The listing builds one solid part. Answer for the finished solid, in the listing's coordinates (mm). A direction names the side the tool comes from. Coordinates: 2 decimals unless noted, no trailing zeros. Write each loop counter-clockwise with the first axis right and the second up, starting at its lowest first coordinate (ties: lowest second). Pieces come first, ordered by that corner, then holes. Notation, with made-up numbers: M 3,80.5 L 53,80.5 A28 cw 53,100.5 Z; hole C 6,-23.5 d5. An arc over 180 degrees is marked long. Answer as CSV lines item,"result".
Autodesk Inventor part; units mm, degrees
ref_plane "YZ Plane" through (0, 0, 0) normal (1, 0, 0) x (0, 1, 0)
ref_plane "XZ Plane" through (0, 0, 0) normal (0, 1, 0) x (-1, 0, 0)
ref_plane "XY Plane" through (0, 0, 0) normal (0, 0, 1) x (1, 0, 0)
sketch "Sketch1" plane through (0, 0, 0) normal (1, 0, 0) x (0, 1, 0)
  line L0 (-4, 6) -> (-4, -6)
  line L1 (-4, -6) -> (-2, -6)
  line L2 (2, -6) -> (4, -6)
  line L3 (4, -6) -> (4, 6)
  line L4 (4, 6) -> (2, 6)
  line L5 (2, 6) -> (0.5, 2)
  line L6 (0.5, 2) -> (-0.5, 2)
  line L7 (-0.5, 2) -> (-2, 6)
  line L8 (-2, 6) -> (-4, 6)
  line L9 (2, -6) -> (0.5, -2)
  line L10 (0.5, -2) -> (-0.5, -2)
  line L11 (-0.5, -2) -> (-2, -6)
  point P0 (0, 0)
  point P1 (-4, 0)
  point P2 (4, 0)
  point P3 (0, 2)
  point P4 (0, -2)
  dimension "d3" = 8
  dimension "d4" = 12
  dimension "d5" = 4
  dimension "d6" = 2
  dimension "d7" = 2
  dimension "d17" = 2
  dimension "d18" = 2
  dimension "d19" = 1
  dimension "d20" = 1
  dimension "d21" = 4
extrude "Extrusion1" add sketch "Sketch1" along normal blind 71
sketch "Sketch2" plane through (0, 4, 6) normal (0, 1, 0) x (1, 0, 0)
  line L0 (0, 12) -> (0, 0)
  point P0 (0, 6)
  point P1 (4, 6)
  point P2 (29, 6)
  point P3 (0, 6)
  point P4 (0, 6)
  point P5 (54, 6)
  dimension "d22" = 4
  dimension "d23" = 25
  dimension "d31" = 25
hole "Hole1" at (4, 4, 0) at (29, 4, 0) at (54, 4, 0) direction (0, -1, 0) diameter 2.459 end through all counterbore diameter 5.5 counterbore depth 3
properties part number "lm_guide_rail" material "Stainless Steel"
Q1. Flat-ended cylindrical pins translate along their axes: pin 1 Ø3 at (x, z) = (29, 0) entering from +Y; pin 2 Ø2 at (x, y) = (55.5, 1.5) entering from -Z; pin 3 Ø2 at (x, z) = (54, 0) entering from -Y. Find the tip coordinate at first contact, or state that the pin passes through.
Output:
pin 1,"y = 1"
pin 2,"z = -6"
pin 3,"through"
Q2. Find section A-A (x = 54). Give the vertices of the cut face in (y, z), and give its area (3 significant figures).
Output:
outline,"M -4,-6 L -2,-6 L -0.5,-2 L 0.5,-2 L 2,-6 L 4,-6 L 4,-2.75 L 1,-2.75 L 1,-1.23 L -4,-1.23 Z; M -4,1.23 L 1,1.23 L 1,2.75 L 4,2.75 L 4,6 L 2,6 L 0.5,2 L -0.5,2 L -2,6 L -4,6 Z"
area,"47.2 mm2"
Q3. Find section B-B (z = 0). Give the vertices of the cut face in (x, y), and give its area (3 significant figures).
Output:
outline,"M 0,-4 L 2.77,-4 L 2.77,1 L 1.25,1 L 1.25,4 L 0,4 Z; M 5.23,-4 L 27.77,-4 L 27.77,1 L 26.25,1 L 26.25,4 L 6.75,4 L 6.75,1 L 5.23,1 Z; M 30.23,-4 L 52.77,-4 L 52.77,1 L 51.25,1 L 51.25,4 L 31.75,4 L 31.75,1 L 30.23,1 Z; M 55.23,-4 L 71,-4 L 71,4 L 56.75,4 L 56.75,1 L 55.23,1 Z"
area,"482 mm2"
Q4. For faces 1 (the flat face through (35, 1.26, 4.03)), 2 (the flat face through (35, 3, 6)), 3 (the flat face through (55, 1, 1)), determine the directions among +Z, -Z, +X, -X, +Y, -Y from which every point of the face is accessible in a straight line to the end or side of a thin tool.
Output:
face 1,"+Z, +X, -X"
face 2,"+Z, +X, -X, +Y, -Y"
face 3,"+Y"
Q5. Find section D-D (x = 27). Give the vertices of the cut face in (y, z).
Output:
outline,"M -4,-6 L -2,-6 L -0.5,-2 L 0.5,-2 L 2,-6 L 4,-6 L 4,-1.89 L 1,-1.89 L 1,1.89 L 4,1.89 L 4,6 L 2,6 L 0.5,2 L -0.5,2 L -2,6 L -4,6 Z"
Q6. Straight lines are drawn through the part: line 1 (X direction, y = 2.1, z = 0); line 2 (X direction, y = -1.05, z = 0); line 3 (Z direction, x = 4, y = -0.1). For each, find the intervals that lie inside material, in ascending order.
Output:
line 1,"0 to 1.25, 6.75 to 26.25, 31.75 to 51.25, 56.75 to 71"
line 2,"0 to 2.77, 5.23 to 27.77, 30.23 to 52.77, 55.23 to 71"
line 3,"-2 to -1.23, 1.23 to 2"
Q7. Find section C-C (z = 5). Give the vertices of the cut face in (x, y) (3 decimals), and give its area (3 significant figures).
Output:
outline,"M 0,-4 L 71,-4 L 71,-1.625 L 0,-1.625 Z; M 0,1.625 L 71,1.625 L 71,4 L 0,4 Z"
area,"337 mm2"
Q8. The mould has two halves that part along Y. Classify faces 4 (the flat face through (35, -1.24, 3.97)), 5 (the flat face through (30, 1, 1)), 6 (the cylindrical face through (52.78, -1.54, -0.16)), 7 (the flat face through (35, -1.24, -3.97)): pulls with the +Y half, pulls with the -Y half, needs draft (parallel to the pull), parting line crosses it, or undercut.
Output:
face 4,"undercut"
face 5,"pulls with the +Y half"
face 6,"needs draft"
face 7,"undercut"
